Build history of the part. All positions in model axes, mm. Give positions to 0.01 mm unless a question says otherwise; leave off trailing zeros. Order: outer loops, then holes, each group sorted by start corner. A loop starts at its lowest first (then second) coordinate and runs counter-clockwise, first axis right, second up. Notation, with made-up numbers: (87, 34) - (105, 34) arc R24 cw to (105, 49) - close; hole circle Ø5 at (56, -1). An arc over 180 degrees is marked (long way). Answer in a Markdown table with one row per item.
```python
from build123d import *

# Parameters (mm, degrees)
SKETCH1_R           = 2.5
BOSS_EXTRUDE1_DEPTH = 8.5
SKETCH3_R           = 2.932976034
BOSS_EXTRUDE3_DEPTH = 1
FILLET1_R           = 2.5
SKETCH4_R           = 0.2
BOSS_EXTRUDE4_DEPTH = 31


with BuildPart() as part:
    # Sketch1 → Boss-Extrude1 (new body)
    with BuildSketch(Plane.XY):
        Circle(SKETCH1_R)
    extrude(amount=BOSS_EXTRUDE1_DEPTH)

    # Sketch3 → Boss-Extrude3 (add)
    with BuildSketch(Plane.XY.offset(8.5)):
        Circle(SKETCH3_R)
    extrude(amount=BOSS_EXTRUDE3_DEPTH)

    # Fillet1
    fillet1_edges = [part.edges().sort_by_distance(p)[0] for p in [
        (-2.5, 0, 0),
    ]]
    fillet(fillet1_edges, radius=FILLET1_R)

    # Sketch4 → Boss-Extrude4 (add)
    with BuildSketch(Plane.XY.offset(9.5)):
        with Locations((-1.71346028, 0)):
            Circle(SKETCH4_R)
        with Locations((-0.44686028, 0)):
            Circle(SKETCH4_R)
        with Locations((0.81979972, 0)):
            Circle(SKETCH4_R)
        with Locations((2.08645972, 0)):
            Circle(SKETCH4_R)
    extrude(amount=BOSS_EXTRUDE4_DEPTH)


solid = part.part
```
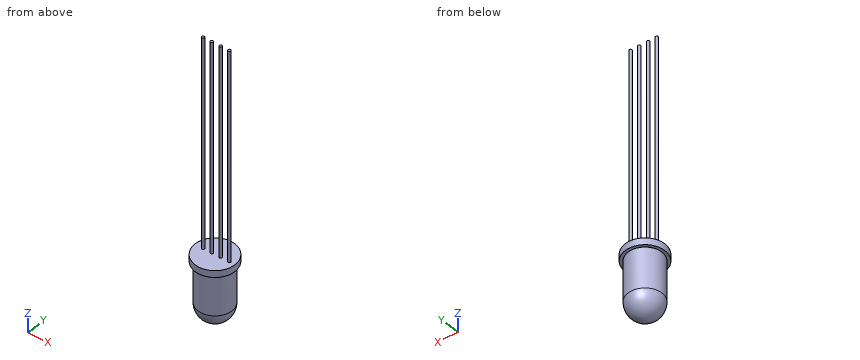
1. Cut at C-C on z = 7. Write the cut outline in (x, y), and give its area (3 significant figures).
Check result:
| item | result |
|---|---|
| outline | circle Ø5 at (0, 0) |
| area | 19.6 mm² |
2. Cut at B-B on y = -0.9. Write the cut outline in (x, z), and give its area (3 significant figures).
Check result:
| item | result |
|---|---|
| outline | (-2.79, 8.5) - (-2.33, 8.5) - (-2.33, 2.5) arc R2.33 ccw to (2.33, 2.5) - (2.33, 8.5) - (2.79, 8.5) - (2.79, 9.5) - (-2.79, 9.5) - close |
| area | 42.1 mm² |
3. Drop flat-ended pins along their axis: P1, Ø2, axis at x = 0, y = 2, coming from the +Z side; P2, Ø3, axis at x = 1.5, z = 26, coming from the +Y side; P3, Ø1.5, axis at x = -1.5, y = -1, coming from the -Z side. Give the stop position or say it passes through.
Check result:
| item | result |
|---|---|
| P1 | stops at z = 9.5 |
| P2 | stops at y = 0.2 |
| P3 | stops at z = 0.23 |
4. Probe line 1 (Y direction, x = 0.85, z = 25.5); line 2 (Z direction, x = -0.7, y = 1.15); line 3 (Z direction, x = -0.5, y = 2.5). List the from-to ranges inside material, lowest first.
Check result:
| item | result |
|---|---|
| line 1 | y = -0.2 to 0.2 |
| line 2 | z = 0.39 to 9.5 |
| line 3 | z = 8.5 to 9.5 |
5. Cut at A-A on z = 37. Write the cut outline in (x, y), and give its area (3 significant figures).
Check result:
| item | result |
|---|---|
| outline | circle Ø0.4 at (-1.71, 0); circle Ø0.4 at (-0.45, 0); circle Ø0.4 at (0.82, 0); circle Ø0.4 at (2.09, 0) |
| area | 0.503 mm² |
